Solid Edge part; units mm, degrees
sketch "Sketch1" plane through (0, 0, 0) normal (0, 0, 1) x (1, 0, 0)
  circle A0 centre (0, 0) radius 3.5
extrude "Protrusion1" add sketch "Sketch1" along normal blind 4
sketch "Sketch2" plane through (0, 0, 4) normal (0, 0, 1) x (0, 1, 0)
  line L0 (0, 1.7321) -> (1.5, 0.866)
  line L1 (1.5, 0.866) -> (1.5, -0.866)
  line L2 (1.5, -0.866) -> (0, -1.7321)
  line L3 (0, -1.7321) -> (-1.5, -0.866)
  line L4 (-1.5, -0.866) -> (-1.5, 0.866)
  line L5 (-1.5, 0.866) -> (0, 1.7321)
extrude "Cutout1" cut sketch "Sketch2" against normal blind 2
fillet "Round1" radius 0.4 1 edges at (-3.5, 0, 4)
sketch "Sketch3" plane through (0, 0, 0) normal (1, 0, 0) x (0, 1, 0)
  line L0 (-1.5705, -12) -> (0, -12)
  line L1 (-2, -11.5705) -> (-1.5705, -12)
  line L2 (-2, -2.1) -> (-2, -11.5705)
  line L3 (-1.5705, -2.1) -> (-2, -2.1)
  line L4 (-1.5705, -2.09) -> (-1.5705, -2.1)
  line L5 (-2, -2.09) -> (-1.5705, -2.09)
  line L6 (-2, -0.2) -> (-2, -2.09)
  arc A0 (-2, -0.2) -> (-2.2, 0) centre (-2.2, -0.2) ccw
revolve "RevolvedProtrusion1" add sketch "Sketch3" angle 360 about axis through (0, 0, -60.325) along (0, 0, 1) material side at (0, -0.7853, -11.95)
cosmetic_thread "Thread1"
sketch "Sketch4" plane through (0, 0, 0) normal (0, -1, 0) x (1, 0, 0)
  line L0 (-1.72, 4) -> (0, 3.007)
revolve "RevolvedCutout1" cut sketch "Sketch4" angle 360 about axis through (0, 0, 57.15) along (0, 0, -1) material side at (-0.835, 0, 3.5468)
properties material "Stahl"
Could you check a few things on this model? Use its own coordinates, in mm. A direction names the side the tool comes from. Round coordinates to 2 decimals unless told otherwise and drop trailing zeros. Write each loop counter-clockwise with the first axis right and the second up, starting at its lowest first coordinate (ties: lowest second). Pieces come first, ordered by that corner, then holes. Notation, with made-up numbers: M -29.75,86 L 21.25,86 A22 ccw 21.25,116 Z; hole C 85.5,84 d6. An arc over 180 degrees is marked long. Answer in a Markdown table with one row per item. Add a question column.
Q1. Will these pins go through, and if not, where does the flat tip stop? pin 1 Ø1.5 at (y, z) = (1, -9) entering from +X; pin 2 Ø1.5 at (x, y) = (0.5, 0.5) entering from +Z; pin 3 Ø3 at (y, z) = (2, -2.5) entering from +X.
Q2. If I drill on line 1 (Y direction, x = -1, z = -5); line 2 (Z direction, x = 2.75, y = -0.75); line 3 (Z direction, x = 0.5, y = 0), over which ranges is the centre line in solid material (lowest first)? Write a range as from..to.
Q3. If we mould it in two halves opening along X, with no side actions, what happens to faces 1 (the flat face through (0, -1.5, 3)), 2 (the flat face through (0, 0, -12)), 3 (the cylindrical face through (2, 0, -7)), 4 (the flat face through (1.293, 0.76, 3.014))? For each: +X half, -X half, draft (parallel to the pull), parting line (faces both ways), or undercut.
Q4. On a 3-axis mill with a long thin cutter (end or side, diameter ignored), from which of +Z, -Z, +X, -X, +Y, -Y can I reach the whole of each face in a straight line? I mean faces 5 (the flat face through (-1.305, 0.74, 3.014)), 6 (the cylindrical face through (3.233, 1.341, 1.775)), 7 (the cylindrical face through (2, 0, -1)). Say none if no direction works.
Q5. Imagine slicing it at B-B (z = -7). Please give me the cut outline in (x, y), then the cut area to 3 significant figures.
Values:
| question | item | result |
|---|---|---|
| 1 | pin 1 | x = 1.98 |
| 1 | pin 2 | z = 2 |
| 1 | pin 3 | x = 1.94 |
| 2 | line 1 | -1.73..1.73 |
| 2 | line 2 | 0..4 |
| 2 | line 3 | -12..2 |
| 3 | face 1 | undercut |
| 3 | face 2 | draft |
| 3 | face 3 | parting line |
| 3 | face 4 | undercut |
| 4 | face 5 | +Z |
| 4 | face 6 | +Z, -Z |
| 4 | face 7 | -Z |
| 5 | outline | C 0,0 d4 |
| 5 | area | 12.6 mm^2 |
